Autodesk Inventor part; units mm, degrees
ref_plane "P2_XY" through (-1, 0, 0) normal (0, -1, 0) x (1, 0, 0)
ref_plane "P2_YZ" through (-1, 0, 0) normal (1, 0, 0) x (0, 0, 1)
ref_plane "P2_ZX" through (-1, 0, 0) normal (0, 0, 1) x (0, -1, 0)
sketch "Sketch_1" plane through (0, 0, 0) normal (1, 0, 0) x (0, 1, 0)
  line L0 (0, 61.9996) -> (0, 0)
  line L1 (0, 0) -> (16.3, 0)
  line L2 (16.3, 0) -> (16.3, 57.632)
  line L3 (16.3, 57.632) -> (0, 61.9996)
extrude "Extrusion1" add sketch "Sketch_1" along normal blind 88
sketch "Sketch_2" plane through (0, 0, 0) normal (0, 0, 1) x (1, 0, 0)
  line L0 (27.5, 20.7) -> (27.5, 12.7)
  line L1 (27.5, 12.7) -> (30.5, 12.7)
  line L2 (30.5, 12.7) -> (30.5, 17.7)
  line L3 (30.5, 17.7) -> (57.5, 17.7)
  line L4 (57.5, 17.7) -> (57.5, 12.7)
  line L5 (57.5, 12.7) -> (60.5, 12.7)
  line L6 (60.5, 12.7) -> (60.5, 20.7)
  line L7 (60.5, 20.7) -> (27.5, 20.7)
extrude "Extrusion2" cut sketch "Sketch_2" along normal blind 65
sketch "Sketch_3" plane through (0, 0, 14.55) normal (0, 0, 1) x (1, 0, 0)
  line L0 (5.575, 27) -> (5.575, 0)
  line L1 (5.575, 0) -> (22.425, 0)
  line L2 (22.425, 0) -> (22.425, 22)
  line L3 (22.425, 22) -> (35.575, 22)
  line L4 (35.575, 22) -> (35.575, 0)
  line L5 (35.575, 0) -> (52.425, 0)
  line L6 (52.425, 0) -> (52.425, 22)
  line L7 (52.425, 22) -> (65.575, 22)
  line L8 (65.575, 22) -> (65.575, 0)
  line L9 (65.575, 0) -> (82.425, 0)
  line L10 (82.425, 0) -> (82.425, 27)
  line L11 (82.425, 27) -> (5.575, 27)
extrude "Extrusion3" cut sketch "Sketch_3" along normal blind 29.2
sketch "Sketch_5" plane through (29, 0, 0) normal (1, 0, 0) x (0, 0, -1)
  line L0 (0, 6.8) -> (-63, 6.8)
  line L1 (-63, 6.8) -> (-63, 10.9)
  line L2 (-63, 10.9) -> (-40, 10.9)
  line L3 (-40, 10.9) -> (-40, 8.9)
  line L4 (-40, 8.9) -> (0, 8.9)
  line L5 (0, 8.9) -> (0, 6.8)
  line L6 (0, 6.8) -> (-63, 6.8)
revolve "Revolution1" cut sketch "Sketch_5" angle 360 about axis through (29, 6.8, 0) along (0, 0, -1)
ref_plane "P2_XY" through (-1, 0, 0) normal (0, -1, 0) x (1, 0, 0)
ref_plane "P2_YZ" through (-1, 0, 0) normal (1, 0, 0) x (0, 0, 1)
ref_plane "P2_ZX" through (-1, 0, 0) normal (0, 0, 1) x (0, -1, 0)
properties part number "nzm1_3p_p2"
Source: CAD feature listing. Evaluate the final solid. Frame: model axes, mm. A direction names the side the tool comes from. Give positions to 0.01 mm unless a question says otherwise; leave off trailing zeros. Order: outer loops, then holes, each group sorted by start corner. A loop starts at its lowest first (then second) coordinate and runs counter-clockwise, first axis right, second up. Notation, with made-up numbers: (70.5, 85) -> (83.5, 85) arc R22 ccw to (83.5, 118) -> close; hole circle Ø5 at (-32.5, -20.5). An arc over 180 degrees is marked (long way). Write item = value, one per line.
Q1. Cut plane A-A, the plane z = 23. Output: boundary loops of the cut face in (x, y) (3 decimals).
Data:
outline = (0, 0) -> (5.575, 0) -> (5.575, 16.3) -> (0, 16.3) -> close; (22.425, 0) -> (35.575, 0) -> (35.575, 16.3) -> (30.5, 16.3) -> (30.5, 12.7) -> (27.5, 12.7) -> (27.5, 16.3) -> (22.425, 16.3) -> close; (52.425, 0) -> (65.575, 0) -> (65.575, 16.3) -> (60.5, 16.3) -> (60.5, 12.7) -> (57.5, 12.7) -> (57.5, 16.3) -> (52.425, 16.3) -> close; (82.425, 0) -> (88, 0) -> (88, 16.3) -> (82.425, 16.3) -> close; hole circle Ø4.2 at (29, 6.8)
Q2. Cut plane D-D, the plane z = 42. Output: boundary loops of the cut face in (x, y) (3 decimals).
Data:
outline = (0, 0) -> (5.575, 0) -> (5.575, 16.3) -> (0, 16.3) -> close; (22.425, 0) -> (35.575, 0) -> (35.575, 16.3) -> (30.5, 16.3) -> (30.5, 12.7) -> (27.5, 12.7) -> (27.5, 16.3) -> (22.425, 16.3) -> close; (52.425, 0) -> (65.575, 0) -> (65.575, 16.3) -> (60.5, 16.3) -> (60.5, 12.7) -> (57.5, 12.7) -> (57.5, 16.3) -> (52.425, 16.3) -> close; (82.425, 0) -> (88, 0) -> (88, 16.3) -> (82.425, 16.3) -> close; hole circle Ø8.2 at (29, 6.8)
Q3. Cut plane C-C, the plane y = 14. Output: boundary loops of the cut face in (x, z) (3 decimals).
Data:
outline = (0, 0) -> (27.5, 0) -> (27.5, 58.248) -> (0, 58.248) -> close; (30.5, 0) -> (57.5, 0) -> (57.5, 58.248) -> (30.5, 58.248) -> close; (60.5, 0) -> (88, 0) -> (88, 58.248) -> (60.5, 58.248) -> close; hole (5.575, 14.55) -> (22.425, 14.55) -> (22.425, 43.75) -> (5.575, 43.75) -> close; hole (35.575, 14.55) -> (52.425, 14.55) -> (52.425, 43.75) -> (35.575, 43.75) -> close; hole (65.575, 14.55) -> (82.425, 14.55) -> (82.425, 43.75) -> (65.575, 43.75) -> close
Q4. Pin query (flat end, axial travel): pin 1 (1 mm diameter, centred on x = 54, z = 27.5, fed in from -Y); pin 2 (2.5 mm diameter, centred on x = 30, y = 7, fed in from +Z); pin 3 (1.5 mm diameter, centred on x = 59, z = 18, fed in from +Y); pin 4 (5 mm diameter, centred on x = 18, y = 11.5, fed in from +Z). Return the tip coordinate at first contact, or that it passes through.
Data:
pin_1 = 0
pin_2 = 40
pin_3 = 12.7
pin_4 = 59.59
Q5. Cut plane B-B, the plane x = 79. Output: boundary loops of the cut face in (y, z), and give its area (3 significant figures).
Data:
outline = (0, 0) -> (16.3, 0) -> (16.3, 14.55) -> (0, 14.55) -> close; (0, 43.75) -> (16.3, 43.75) -> (16.3, 57.63) -> (0, 62) -> close
area = 499 mm^2
Q6. Pull-direction query (X, two-part tool) for faces 6 (the face through (88, 8, 31)), 7 (the face through (34, 0, 31)), 8 (the face through (0, 8, 31)), 9 (the face through (27.137, 7.769, 19.72)); classes: released by +X, released by -X, zero draft, split by the parting line, or undercut.
Data:
face_6 = released by +X
face_7 = zero draft
face_8 = released by -X
face_9 = undercut
Q7. Set-up query: faces 1 (the face through (29, 12.7, 29)), 2 (the face through (27, 9, 40)), 3 (the face through (35, 16.3, 28)), 4 (the face through (43, 8, 0)), 5 (the face through (14, 8, 43.75)). Return all of +Z, -Z, +X, -X, +Y, -Y with unobstructed straight access to the full face (end or side cutting, diameter ignored); none if empty.
Data:
face_1 = +Z, -Z, +Y
face_2 = +Z
face_3 = +Z, -Z, +X, -X, +Y
face_4 = -Z, +X, -X, +Y, -Y
face_5 = +Y, -Y
Q8. Material intervals for line 1 (X direction, y = 6.8, z = 22.5) (3 decimals); line 2 (X direction, y = 6.8, z = 52.75); line 3 (Y direction, x = 29, z = 45.25), sorted ascending. Write a range as from..to.
Data:
line_1 = 0..5.575, 22.425..26.9, 31.1..35.575, 52.425..65.575, 82.425..88
line_2 = 0..24.9, 33.1..88
line_3 = 0..2.7, 10.9..12.7
